```python
from build123d import *

# Parameters (mm, degrees)
EXTRUDE_1_DEPTH     = 5
EXTRUDE_2_DEPTH     = 13
EXTRUDE_3_DEPTH     = 10
EXTRUDE_4_DEPTH     = 7.28
EXTRUDE_START       = -9.8
EXTRUDE_5_DEPTH     = 4.8
SKETCH_2_23_R       = 1.225
CUT_EXTRUDE_1_DEPTH = 5


# Read off the part's stored shape, not the designer's step: the extrude step
with BuildPart() as part:
    # Sketch 2 → Extrude 1 (new body)
    with BuildSketch(Plane(origin=(0, 0, 0), x_dir=(1, 0, 0), z_dir=(0, 1, 0))):
        with BuildLine():
            Line((69.8, -1.428456646), (69.8, -66.428456646))
            ThreePointArc((69.8, -66.428456646), (68.39411255, -69.822569196), (65, -71.228456646))
            Line((65, -71.228456646), (-65, -71.228456646))
            ThreePointArc((-65, -71.228456646), (-68.39411255, -69.822569196), (-69.8, -66.428456646))
            Line((-69.8, -66.428456646), (-69.8, -1.428456646))
            ThreePointArc((-69.8, -1.428456646), (-68.39411255, 1.965655904), (-65, 3.371543354))
            Line((-65, 3.371543354), (65, 3.371543354))
            ThreePointArc((65, 3.371543354), (68.39411255, 1.965655904), (69.8, -1.428456646))
        make_face()
    extrude(amount=-EXTRUDE_1_DEPTH)

    # Sketch 2_19 → Extrude 2 (add)
    with BuildSketch(Plane(origin=(0, 0, 0), x_dir=(1, 0, 0), z_dir=(0, 1, 0))):
        Polygon((14.518227689, -71.177974158), (-3.231616409, -46.992378558), (-10.358382401, -52.222722576), (-10.358382401, -57.563452802), (-0.32961603, -71.228456646), (5.748381901, -71.228456646), (-6.056399498, -55.143488942), (-4.282789154, -53.841833708), (7.668772538, -70.126801412), (8.477278931, -71.228456646), (14.555276861, -71.228456646), align=None)
    extrude(amount=-EXTRUDE_2_DEPTH)

    # Sketch 2_20 → Extrude 3 (add)
    with BuildSketch(Plane(origin=(0, 0, 0), x_dir=(1, 0, 0), z_dir=(0, 1, 0))):
        Polygon((39.164167684, -2.982298959), (57.842076132, -60.001030407), (41.971862546, -65.199714925), (23.293954098, -8.180983477), align=None)
        Polygon((36.033000472, -9.164191217), (29.475846356, -11.312150688), (45.103029757, -59.017822667), (51.660183874, -56.869863196), align=None, mode=Mode.SUBTRACT)
    extrude(amount=-EXTRUDE_3_DEPTH)

    # Sketch 2_21 → Extrude 4 (add)
    with BuildSketch(Plane(origin=(0, 0, 0), x_dir=(1, 0, 0), z_dir=(0, 1, 0))):
        Polygon((36.033000472, -9.164191217), (51.660183874, -56.869863196), (45.103029757, -59.017822667), (29.475846356, -11.312150688), align=None)
    extrude(amount=-EXTRUDE_4_DEPTH)

    # Extrude 5 outline → Extrude 5 (add)
    with BuildSketch(Plane(origin=(0, 0, 0), x_dir=(1, 0, 0), z_dir=(0, 1, 0)).offset(EXTRUDE_START)):
        Polygon((5.748381901, -71.228456646), (8.477278931, -71.228456646), (-4.282789154, -53.841833708), (-6.056399498, -55.143488942), align=None)
    extrude(amount=EXTRUDE_5_DEPTH)

    # Sketch 2_23 → Cut-Extrude 1 (cut)
    with BuildSketch(Plane(origin=(0, 0, 0), x_dir=(1, 0, 0), z_dir=(0, 1, 0))):
        with Locations(Location((-65, -1.428456646, 0), (0, 0, 270))):
            Circle(SKETCH_2_23_R)
        with Locations(Location((-65, -66.428456646, 0), (0, 0, 270))):
            Circle(SKETCH_2_23_R)
        with Locations(Location((65, -66.428456646, 0), (0, 0, 270))):
            Circle(SKETCH_2_23_R)
        with Locations(Location((65, -1.428456646, 0), (0, 0, 270))):
            Circle(SKETCH_2_23_R)
    extrude(amount=-CUT_EXTRUDE_1_DEPTH, mode=Mode.SUBTRACT)


solid = part.part
```
Verification items for the finished model (mm, model axes). A direction names the side the tool comes from. Give positions to 0.01 mm unless a question says otherwise; leave off trailing zeros. Loops run counter-clockwise (first coordinate to the right, second up) from the corner with the lowest first, then second, coordinate; pieces in that order, holes last. Notation, with made-up numbers: M 37,74 L 45,74 A19 cw 45,91 Z; hole C 57,25 d2. An arc over 180 degrees is marked long. Return JSON: item names as keys, results as strings.
1) Gauge pin test, flat ends, axial feed: P1, Ø4, axis at y = -10, z = 41, coming from the +X side; P2, Ø4, axis at x = 65, z = 66.43, coming from the -Y side; P3, Ø1.6, axis at y = -9, z = 53.5, coming from the -X side. Record the tip position at first contact, or that the pin passes through.
Findings:
{"P1": "stops at x = 52.27", "P2": "stops at y = -5", "P3": "stops at x = -10.36"}
2) Mould release check, pull along X, two halves, no side actions. Record for faces 5 (the cylindrical face through (-68.357, -2.465, 69.86)), 6 (the cylindrical face through (66.03, -2.46, 2.09)), 7 (the flat face through (38, -10, 39)), 8 (the cylindrical face through (68.431, -2.465, 69.785)): released by +X, released by -X, zero draft, split by the parting line, or undercut.
Findings:
{"face 5": "released by -X", "face 6": "undercut", "face 7": "zero draft", "face 8": "released by +X"}
3) Material ranges on L1, parallel to Z at x = -65, y = -1.2; L2, parallel to X at y = -8.25, z = 51; L3, parallel to X at y = -2.75, z = 2, recorded low to high. Write a range as [from, to].
Findings:
{"L1": "z = [-3.37, 0.2], [2.65, 65.2], [67.65, 71.23]", "L2": "x = [-8.69, -0.29], [37.32, 42.48], [49.74, 54.89]", "L3": "x = [-69.8, -66.08], [-63.92, 63.92], [66.08, 69.8]"}
4) Section check A-A, the plane x = -47. Enter the section's corners in (y, z).
Findings:
{"outline": "M -5,-3.37 L 0,-3.37 L 0,71.23 L -5,71.23 Z"}
5) Section check B-B, the plane z = 63. Enter the section's corners in (x, y), and give its area (3 significant figures).
Findings:
{"outline": "M -69.8,-5 L -6.37,-5 L -6.37,-13 L -0.29,-13 L -0.29,-9.8 L 2.44,-9.8 L 2.44,-13 L 8.52,-13 L 8.52,-5 L 41.25,-5 L 41.25,-10 L 48.69,-10 L 48.69,-5 L 69.8,-5 L 69.8,0 L -69.8,0 Z", "area": "846 mm2"}
6) Tool access check on faces 1 (the flat face through (48.37, -7.46, 31.09)), 2 (the flat face through (43.956, -8.621, 33.351)), 3 (the flat face through (-5.414, -8.944, 64.3)), 4 (the flat face through (50.018, -7.465, 62.564)). Record the directions out of +Z, -Z, +X, -X, +Y, -Y that give a thin tool (end or side, any length) a straight path to the whole face; none if there is none.
Findings:
{"face 1": "-Z, +X, -Y", "face 2": "-Y", "face 3": "+Z, -X, -Y", "face 4": "+Z, +X, -Y"}
7) Section check C-C, the plane x = 34.5. Enter the section's corners in (y, z), and give its area (3 significant figures).
Findings:
{"outline": "M -10,4.51 L -5,4.51 L -5,-3.37 L 0,-3.37 L 0,71.23 L -5,71.23 L -5,42.39 L -10,42.39 L -10,26.65 L -7.28,26.65 L -7.28,9.67 L -10,9.67 Z", "area": "516 mm2"}
